```python
from build123d import *

# Parameters (mm, degrees)
F0_R     = 25.4
F0_R_2   = 3.81
F1_DEPTH = 12.7


with BuildPart() as f1:
    # F0 (on Top) → F1 (new body)
    with BuildSketch(Plane.XY):
        Circle(F0_R)
        with BuildLine():
            Line((-17.78, 0), (17.78, 0))
            ThreePointArc((17.78, 0), (0, -17.78), (-17.78, 0))
        make_face(mode=Mode.SUBTRACT)
        with Locations((-7.62, 12.7)):
            Circle(F0_R_2, mode=Mode.SUBTRACT)
        with Locations((7.62, 12.7)):
            Circle(F0_R_2, mode=Mode.SUBTRACT)
    extrude(amount=F1_DEPTH)


solid = f1.part
```
Here's how the part is built. I have some questions about the finished solid (model axes, mm). A direction names the side the tool comes from. Round coordinates to 2 decimals unless told otherwise and drop trailing zeros. Order: outer loops, then holes, each group sorted by start corner. A loop starts at its lowest first (then second) coordinate and runs counter-clockwise, first axis right, second up. Notation, with made-up numbers: M 71.25,-26.75 L 119.25,-26.75 A15 ccw 119.25,-20.75 Z; hole C -14,-10.5 d2. An arc over 180 degrees is marked long. Answer as CSV lines item,"result".
Item 1: We'd pull the mould along X, two halves only. Please class faces 1 (the cylindrical face through (-4.1, 11.24, 6.26)), 2 (the flat face through (-0.4, 0.4, 0)), 3 (the cylindrical face through (-5.506, -24.796, 6.261)): +X half, -X half, draft (parallel to the pull), parting line (faces both ways), or undercut.
From the geometry:
face 1,"undercut"
face 2,"draft"
face 3,"parting line"
Item 2: Imagine slicing it at C-C on y = -5.5. List the corners of the cut face in (x, z) for me.
From the geometry:
outline,"M -24.8,0 L -16.91,0 L -16.91,12.7 L -24.8,12.7 Z; M 16.91,0 L 24.8,0 L 24.8,12.7 L 16.91,12.7 Z"
Item 3: Please list where these lines run through material, in increasing order: L1, parallel to Y at x = 7.62, z = 4.5; L2, parallel to Y at x = 10.5, z = 12; L3, parallel to Y at x = -2.5, z = 3. Write a range as [from, to].
From the geometry:
L1,"[-24.23, -16.06], [0, 8.89], [16.51, 24.23]"
L2,"[-23.13, -14.35], [0, 10.21], [15.19, 23.13]"
L3,"[-25.28, -17.6], [0, 25.28]"
Item 4: For pin 1 (6 mm diameter, centred on x = -10.5, z = 7.5, fed in from -Y); pin 2 (5 mm diameter, centred on y = -7.5, z = 8.5, fed in from +X); pin 3 (6.5 mm diameter, centred on x = 9, z = 8, fed in from -Y), each with a flat end and sliding along its axis, tell me the tip position at first contact or that it passes through.
From the geometry:
pin 1,"y = -24.27"
pin 2,"x = 24.9"
pin 3,"y = -24.74"
Item 5: Imagine slicing it at B-B on z = 6.25. List the corners of the cut face in (x, y) for me.
From the geometry:
outline,"C 0,0 d50.8; hole M -17.78,0 A17.78 ccw 17.78,0 Z; hole C -7.62,12.7 d7.62; hole C 7.62,12.7 d7.62"
Item 6: Imagine slicing it at D-D on x = 7.62. List the corners of the cut face in (y, z) for me.
From the geometry:
outline,"M -24.23,0 L -16.06,0 L -16.06,12.7 L -24.23,12.7 Z; M 0,0 L 8.89,0 L 8.89,12.7 L 0,12.7 Z; M 16.51,0 L 24.23,0 L 24.23,12.7 L 16.51,12.7 Z"
Item 7: Imagine slicing it at A-A on x = 0. List the corners of the cut face in (y, z) for me, and give its area (3 significant figures).
From the geometry:
outline,"M -25.4,0 L -17.78,0 L -17.78,12.7 L -25.4,12.7 Z; M 0,0 L 25.4,0 L 25.4,12.7 L 0,12.7 Z"
area,"419 mm2"
Item 8: Which directions (+Z, -Z, +X, -X, +Y, -Y) give clear straight access to the entire face, cutting with the end or side of a thin tool? Please do faces 4 (the flat face through (-0.4, 0.4, 12.7)), 5 (the flat face through (0, 0, 6)).
From the geometry:
face 4,"+Z, +X, -X, +Y, -Y"
face 5,"+Z, -Z"
